For this review, take the finished solid that the model builds, in its own axes (mm). A direction names the side the tool comes from. Coordinates: 2 decimals unless noted, no trailing zeros. Order: outer loops, then holes, each group sorted by start corner. A loop starts at its lowest first (then second) coordinate and runs counter-clockwise, first axis right, second up. Notation, with made-up numbers: (49, 14.5) -> (59, 14.5) arc R24 ccw to (59, 45.5) -> close; hole circle Ø11 at (21.5, 34). An arc over 180 degrees is marked (long way). Write item = value, one per line. Start each with the question number.
1) Consider section C-C on z = 4. Give the boundary of the cut face in (x, y).
2) Wall thickness on probe 1 along X at (y, z) = (-22, 17); probe 2 along Z at (x, y) = (32.5, -21.5); probe 3 along Z at (x, y) = (-42.5, -35.5): over which ranges is each line inside the solid? List them lowest first. Write a range as [from, to].
3) Consider section A-A on y = -13.5. Give the boundary of the cut face in (x, z), and give its area (3 significant figures).
4) Machinability: for faces 1 (the face through (25, -20, 17)), 2 (the face through (-25, -20, 12)), 3 (the face through (50, -20, -13)), which of the approach directions +Z, -Z, +X, -X, +Y, -Y give a long, thin tool a straight path to every point of the face, cutting with its end or side? Answer none if there is none.
5) Insertion check: pin 1 Ø6 at (y, z) = (-11.5, 9) entering from +X; pin 2 Ø5 at (y, z) = (-28.5, 1) entering from -X; pin 3 Ø12.5 at (x, y) = (-42.5, -24) entering from +Z. Each pin has a flat end and moves straight along its axis. Give the tip position at first contact, or say it passes through.
6) Consider section B-B on x = 42. Give the boundary of the cut face in (y, z).
from build123d import *

# Parameters (mm, degrees)
F0_W     = 100
F0_H     = 60
F1_DEPTH = 40
F2_W     = 25
F2_H     = 35
F2_H_2   = 25
F3_DEPTH = 40.001


with BuildPart() as f1:
    # F0 (on Front) → F1 (new body)
    with BuildSketch(Plane.XZ):
        Rectangle(F0_W, F0_H)
    extrude(amount=F1_DEPTH)

    # F2 (on face) → F3 (cut, through all)
    with BuildSketch(Plane.XZ.offset(40)):
        with Locations((-37.5, 12.5)):
            Rectangle(F2_W, F2_H)
        with Locations((37.5, 17.5)):
            Rectangle(F2_W, F2_H_2)
    extrude(amount=-F3_DEPTH, mode=Mode.SUBTRACT)


solid = f1.part
Answer sheet:
q1.outline = (-25, -40) -> (50, -40) -> (50, 0) -> (-25, 0) -> close
q2.probe_1 = [-25, 25]
q2.probe_2 = [-30, 5]
q2.probe_3 = [-30, -5]
q3.outline = (-50, -30) -> (50, -30) -> (50, 5) -> (25, 5) -> (25, 30) -> (-25, 30) -> (-25, -5) -> (-50, -5) -> close
q3.area = 4,500 mm2
q4.face_1 = +Z, +X, +Y, -Y
q4.face_2 = +Z, -X, +Y, -Y
q4.face_3 = +Z, -Z, +X, +Y, -Y
q5.pin_1 = 25
q5.pin_2 = -25
q5.pin_3 = -5
q6.outline = (-40, -30) -> (0, -30) -> (0, 5) -> (-40, 5) -> close
